from build123d import *

# Parameters (mm, degrees)
REVOLUTION_ANGLE      = 180
SKETCH001_R           = 2.5
POCKET_DEPTH          = 20
POLARPATTERN_COUNT    = 6
POLARPATTERN_ANGLE    = 150
SKETCH002_R           = 1
POCKET001_DEPTH       = 5
POLARPATTERN001_COUNT = 10
SKETCH003_R           = 1
POCKET002_DEPTH       = 5
POLARPATTERN002_COUNT = 10
SKETCH004_R           = 2.5
POCKET003_DEPTH       = 5
POLARPATTERN003_COUNT = 10
SKETCH005_R           = 3
POCKET004_DEPTH       = 5
POLARPATTERN004_COUNT = 10
LINEARPATTERN_COUNT   = 10
LINEARPATTERN_PITCH   = 0.555556


with BuildPart() as part:
    # Sketch → Revolution (revolve)
    with BuildSketch(Plane.XY):
        Polygon((-37.5, 0), (-37.5, 7), (-32.5, 7), (-32.5, 17), (-30, 17), (-30, 7), (20, 7), (20, 25.4), (22.5, 25.4), (22.5, 17.5), (28.5, 17.5), (28.5, 16.4), (32.5, 16.4), (32.5, 7), (37.5, 7), (37.5, 0), align=None)
    revolve(axis=Axis((0, 0, 0), (1, 0, 0)), revolution_arc=REVOLUTION_ANGLE)

    # Sketch001 → Pocket (cut)
    with BuildSketch(Plane.YZ.offset(32.5)):
        with Locations((-11.128845, 3.166362)):
            Circle(SKETCH001_R)
    pocket = extrude(amount=-POCKET_DEPTH, mode=Mode.SUBTRACT)

    # PolarPattern: Pocket ×6 about axis
    polarpattern_axis = Axis((32.5, 0, 0), (-1, 0, 0))
    for i in range(1, POLARPATTERN_COUNT):
        add(pocket.rotate(polarpattern_axis, i * POLARPATTERN_ANGLE / (POLARPATTERN_COUNT - 1)), mode=Mode.SUBTRACT)

    # Sketch002 → Pocket001 (cut)
    with BuildSketch(Plane(origin=(-32.5, 0, 0), x_dir=(0, -1, 0), z_dir=(-1, 0, 0))):
        with Locations((-14.077337, 0)):
            Circle(SKETCH002_R)
    pocket001 = extrude(amount=-POCKET001_DEPTH, mode=Mode.SUBTRACT)

    # PolarPattern001: Pocket001 ×10 about axis
    polarpattern001_axis = Axis((-32.5, 0, 0), (-1, 0, 0))
    for i in range(1, POLARPATTERN001_COUNT):
        add(pocket001.rotate(polarpattern001_axis, i * 360 / POLARPATTERN001_COUNT), mode=Mode.SUBTRACT)

    # Sketch003 → Pocket002 (cut)
    with BuildSketch(Plane(origin=(20, 0, 0), x_dir=(0, -1, 0), z_dir=(-1, 0, 0))):
        with Locations((-21.398772, 6.952882)):
            Circle(SKETCH003_R)
    pocket002 = extrude(amount=-POCKET002_DEPTH, mode=Mode.SUBTRACT)

    # PolarPattern002: Pocket002 ×10 about axis
    polarpattern002_axis = Axis((20, 0, 0), (-1, 0, 0))
    for i in range(1, POLARPATTERN002_COUNT):
        add(pocket002.rotate(polarpattern002_axis, i * 360 / POLARPATTERN002_COUNT), mode=Mode.SUBTRACT)

    # Sketch004 → Pocket003 (cut)
    with BuildSketch(Plane(origin=(-32.5, 0, 0), x_dir=(0, -1, 0), z_dir=(-1, 0, 0))):
        with Locations((-10.461622, 3.399187)):
            Circle(SKETCH004_R)
    pocket003 = extrude(amount=-POCKET003_DEPTH, mode=Mode.SUBTRACT)

    # PolarPattern003: Pocket003 ×10 about axis
    polarpattern003_axis = Axis((-32.5, 0, 0), (-1, 0, 0))
    for i in range(1, POLARPATTERN003_COUNT):
        add(pocket003.rotate(polarpattern003_axis, i * 360 / POLARPATTERN003_COUNT), mode=Mode.SUBTRACT)

    # Sketch005 → Pocket004 (cut)
    with BuildSketch(Plane(origin=(20, 0, 0), x_dir=(0, -1, 0), z_dir=(-1, 0, 0))):
        with Locations((-21, 0)):
            Circle(SKETCH005_R)
    pocket004 = extrude(amount=-POCKET004_DEPTH, mode=Mode.SUBTRACT)

    # PolarPattern004: Pocket004 ×10 about axis
    polarpattern004_axis = Axis((20, 0, 0), (-1, 0, 0))
    for i in range(1, POLARPATTERN004_COUNT):
        add(pocket004.rotate(polarpattern004_axis, i * 360 / POLARPATTERN004_COUNT), mode=Mode.SUBTRACT)

    # Sketch006 → Groove (revolve, cut)
    with BuildSketch(Plane(origin=(0, 0, 0), x_dir=(1, 0, 0), z_dir=(0, 0, -1))):
        Polygon((22.586137, 17.633119), (22.85774, 17.162689), (23.109543, 17.598824), (23.109543, 18.335896), (22.603432, 18.335896), align=None)
    groove = revolve(axis=Axis((0, 0, 0), (1, 0, 0)), mode=Mode.SUBTRACT)

    # LinearPattern: Groove ×10
    with Locations(*[(i * LINEARPATTERN_PITCH, 0, 0) for i in range(1, LINEARPATTERN_COUNT)]):
        add(groove, mode=Mode.SUBTRACT)


solid = part.part
Part model, mm, in its own coordinate system. A direction names the side the tool comes from. Give positions to 0.01 mm unless a question says otherwise; leave off trailing zeros. Order: outer loops, then holes, each group sorted by start corner. A loop starts at its lowest first (then second) coordinate and runs counter-clockwise, first axis right, second up. Notation, with made-up numbers: (11, 70.25) -> (67, 70.25) arc R14 cw to (67, 96.25) -> close; hole circle Ø4 at (1.5, 30). An arc over 180 degrees is marked (long way). Use one line per item in the form item = value.
(1) Saw through at B-B (z = 4.25). Count the separate pieces of the cut face and the enclosed holes in it, then the cut area to 3 significant figures.
Solution:
separate_pieces = 5
enclosed_holes = 0
area = 1,070 mm²
(2) Drill centre lines: line 1 (X direction, y = -13, z = 10.75); line 2 (X direction, y = -1, z = 8.5); line 3 (Z direction, x = 22, y = 4). Where is each one in solid material? Low to high. Write a range as from..to.
Solution:
line_1 = -32.5..-30, 20..28.5
line_2 = -32.5..-30, 20..32.5
line_3 = 0..8.77, 13.49..18.3, 21.65..25.08
(3) Saw through at A-A (x = -2.5). Write the cut outline in (y, z), then the cut area to 3 significant figures.
Solution:
outline = (-7, 0) -> (7, 0) arc R7 ccw to start
area = 77.0 mm²
(4) Tool access for faces 4 (the face through (21.23, 19.99, 12.27)), 5 (the face through (-31, 0, 17)), 6 (the face through (-31.27, 12.96, 3.51)): list every direction of +Z, -Z, +X, -X, +Y, -Y with a clear straight run to the whole face (end or side of a thin tool).
Solution:
face_4 = +X, -X
face_5 = +Z, -X
face_6 = -X
(5) Pull direction X, two halves, no side cores. Call faces 1 (the face through (25.54, 0.38, 17.32)), 2 (the face through (-31.268, -10.794, 7.471)), 3 (the face through (-32.5, 4, 7)): +X half, -X half, draft (parallel to the pull), parting line (faces both ways), or undercut.
Solution:
face_1 = undercut
face_2 = draft
face_3 = -X half
(6) Flat gauge pins, fed straight in: P1, Ø6, axis at y = -6.47, z = 8.9, coming from the -X side; P2, Ø2.5, axis at y = 0, z = 22.5, coming from the -X side; P3, Ø5, axis at x = 5, y = -5.5, coming from the +Z side; P4, Ø5, axis at y = -6, z = 6, coming from the -X side. Where does each tip first touch, or does it go through?
Solution:
P1 = -32.5
P2 = 20
P3 = 6.32
P4 = -37.5
